```python
from build123d import *

# Parameters (mm, degrees)
ESQUISSE1_W             = 80
ESQUISSE1_H             = 80
BOSS_EXTRU_1_DEPTH      = 25
ESQUISSE2_W             = 76.4
ESQUISSE2_H             = 76.4
ENL_V_MAT_EXTRU_3_DEPTH = 22
ESQUISSE3_W             = 10
ESQUISSE3_H             = 15
ESQUISSE3_H_2           = 10
BOSS_EXTRU_2_DEPTH      = 9
ESQUISSE4_W             = 10
ESQUISSE4_H             = 10.9
ESQUISSE4_W_2           = 6
ESQUISSE4_H_2           = 10
BOSS_EXTRU_3_DEPTH      = 4
ESQUISSE5_W             = 11.2
ESQUISSE5_H             = 9.2
ESQUISSE5_W_2           = 6
ESQUISSE5_H_2           = 10.5
ENL_V_MAT_EXTRU_4_DEPTH = 10
CONG_2_R                = 2
CONG_3_R                = 1
ENL_V_MAT_EXTRU_5_DEPTH = 0.5
ENL_V_MAT_EXTRU_6_DEPTH = 0.5
ENL_V_MAT_EXTRU_7_DEPTH = 2
ENL_V_START             = -2
ENL_V_MAT_EXTRU_8_DEPTH = 2


with BuildPart() as part:
    # Esquisse1 → Boss.-Extru.1 (new body)
    with BuildSketch(Plane.XY):
        with Locations((40, 40)):
            Rectangle(ESQUISSE1_W, ESQUISSE1_H)
    extrude(amount=BOSS_EXTRU_1_DEPTH)

    # Esquisse2 → Enlèv. mat.-Extru.3 (cut)
    with BuildSketch(Plane.XY.offset(25)):
        with Locations((40.2, 40.2)):
            Rectangle(ESQUISSE2_W, ESQUISSE2_H)
    extrude(amount=-ENL_V_MAT_EXTRU_3_DEPTH, mode=Mode.SUBTRACT)

    # Esquisse3 → Boss.-Extru.2 (add)
    with BuildSketch(Plane.XY.offset(3)):
        with Locations((20, 9.5)):
            Rectangle(ESQUISSE3_W, ESQUISSE3_H)
        with Locations((73.4, 39.688534772)):
            Rectangle(ESQUISSE3_W, ESQUISSE3_H_2)
        with Locations((20, 70.9)):
            Rectangle(ESQUISSE3_W, ESQUISSE3_H)
    extrude(amount=BOSS_EXTRU_2_DEPTH)

    # Esquisse4 → Boss.-Extru.3 (add)
    with BuildSketch(Plane.XY.offset(12)):
        with Locations((20, 7.45)):
            Rectangle(ESQUISSE4_W, ESQUISSE4_H)
        with Locations((20, 72.95)):
            Rectangle(ESQUISSE4_W, ESQUISSE4_H)
        with Locations((75.4, 39.688534772)):
            Rectangle(ESQUISSE4_W_2, ESQUISSE4_H_2)
    extrude(amount=BOSS_EXTRU_3_DEPTH)

    # Esquisse5 → Enlèv. mat.-Extru.4 (cut)
    with BuildSketch(Plane.ZY):
        with Locations((19.4, 21)):
            Rectangle(ESQUISSE5_W, ESQUISSE5_H)
        with Locations((15, 33.25)):
            Rectangle(ESQUISSE5_W_2, ESQUISSE5_H_2)
    extrude(amount=-ENL_V_MAT_EXTRU_4_DEPTH, mode=Mode.SUBTRACT)

    # Congé2
    cong_2_edges = [part.edges().sort_by_distance(p)[0] for p in [
        (1, 28, 12),
        (1, 38.5, 12),
    ]]
    fillet(cong_2_edges, radius=CONG_2_R)

    # Congé3
    cong_3_edges = [part.edges().sort_by_distance(p)[0] for p in [
        (1, 38.5, 18),
        (1, 28, 18),
    ]]
    fillet(cong_3_edges, radius=CONG_3_R)

    # Esquisse8 → Enlèv. mat.-Extru.5 (cut)
    with BuildSketch(Plane.ZY):
        with BuildLine():
            add(Edge.make_bspline(
                [(7.313237468, 65.833159363), (7.48897389, 65.712447359), (7.804126252, 65.49597161), (8.487346274, 65.283616184), (8.981094379, 65.226001547), (9.307707678, 65.18788959)],
                knots=[0, 0, 0, 0, 0.299076085, 0.536340353, 1, 1, 1, 1], degree=3))
            add(Edge.make_bspline(
                [(7.284702647, 65.80245585), (7.293856567, 65.81317431), (7.303547017, 65.823166837), (7.313237468, 65.833159363)],
                knots=[0.816445355, 0.816445355, 0.816445355, 0.816445355, 1, 1, 1, 1], degree=3))
            add(Edge.make_bspline(
                [(17.901527847, 50.874632789), (17.356129628, 51.530826995), (16.293469748, 52.809362994), (15.275532925, 55.228252674), (13.933854466, 57.885340246), (11.93358483, 60.745765414), (9.727873266, 63.52670077), (8.030552607, 65.116137898), (7.284702647, 65.80245585)],
                knots=[0, 0, 0, 0, 0.134488449, 0.262038771, 0.413324325, 0.606278792, 0.814215894, 0.974718857, 0.974718857, 0.974718857, 0.974718857], degree=3))
            add(Edge.make_bspline(
                [(7.407085151, 65.469076199), (7.997724667, 64.952415937), (9.572762834, 63.532102924), (11.741354127, 60.845320938), (13.846315376, 57.844082794), (15.265007359, 55.100127721), (16.333677342, 52.722721211), (17.367018575, 51.504680356), (17.901527847, 50.874632789)],
                knots=[0.043476968, 0.043476968, 0.043476968, 0.043476968, 0.167785205, 0.379770977, 0.589080615, 0.748039182, 0.869669971, 1, 1, 1, 1], degree=3))
            add(Edge.make_bspline(
                [(7.987837686, 63.516054267), (7.933705658, 63.852405499), (7.85098554, 64.366389832), (7.741769984, 65.069503506), (7.523361561, 65.343113704), (7.407085151, 65.469076199)],
                knots=[0, 0, 0, 0, 0.449393835, 0.686726756, 0.906490115, 0.906490115, 0.906490115, 0.906490115], degree=3))
            add(Edge.make_bspline(
                [(9.581947331, 60.333994368), (9.35896114, 60.695257019), (8.925646923, 61.397274669), (8.371533969, 62.453225866), (8.111622296, 63.17317422), (7.987837686, 63.516054267)],
                knots=[0, 0, 0, 0, 0.357022344, 0.693777745, 1, 1, 1, 1], degree=3))
            add(Edge.make_bspline(
                [(9.923647007, 61.990871165), (9.797152593, 61.702831345), (9.59150409, 61.234550131), (9.533644523, 60.653068807), (9.572467818, 60.3966133), (9.581947331, 60.333994368)],
                knots=[0, 0, 0, 0, 0.547075637, 0.889409121, 1, 1, 1, 1], degree=3))
            add(Edge.make_bspline(
                [(9.845334721, 59.996400955), (9.811598018, 60.115915835), (9.717723572, 60.448473327), (9.824688072, 61.125443291), (9.886572886, 61.666645995), (9.923647007, 61.990871165)],
                knots=[0, 0, 0, 0, 0.183614026, 0.510917298, 1, 1, 1, 1], degree=3))
            add(Edge.make_bspline(
                [(12.516751585, 56.360012475), (12.220146813, 56.731946706), (11.602008437, 57.507075242), (10.696458869, 58.709807691), (10.128597293, 59.568209935), (9.845334721, 59.996400955)],
                knots=[0, 0, 0, 0, 0.316155138, 0.658882265, 1, 1, 1, 1], degree=3))
            add(Edge.make_bspline(
                [(12.5243775, 58.549530139), (12.475747631, 58.195383202), (12.389698733, 57.568732254), (12.460969789, 56.835777723), (12.504804941, 56.461905897), (12.516751585, 56.360012475)],
                knots=[0, 0, 0, 0, 0.485970736, 0.859908672, 1, 1, 1, 1], degree=3))
            add(Edge.make_bspline(
                [(12.712972257, 56.117743005), (12.689100366, 56.22919998), (12.605595842, 56.619079516), (12.538586692, 57.433441747), (12.529671109, 58.133733427), (12.5243775, 58.549530139)],
                knots=[0, 0, 0, 0, 0.139880518, 0.489305866, 1, 1, 1, 1], degree=3))
            add(Edge.make_bspline(
                [(13.853926539, 54.716920987), (13.770782279, 54.821999659), (13.560207416, 55.088126596), (13.175056735, 55.551153097), (12.879119476, 55.914019785), (12.712972257, 56.117743005)],
                knots=[0, 0, 0, 0, 0.222488299, 0.563483801, 1, 1, 1, 1], degree=3))
            add(Edge.make_bspline(
                [(18.605458509, 50.170702126), (18.280931893, 50.44303874), (17.255771256, 51.303334203), (15.614574097, 52.765406202), (14.427661827, 54.080988547), (13.853926539, 54.716920987)],
                knots=[0, 0, 0, 0, 0.193087, 0.609950563, 1, 1, 1, 1], degree=3))
            add(Edge.make_bspline(
                [(16.20036208, 54.159642546), (16.438779976, 53.603827531), (16.879859527, 52.575554733), (17.742560122, 51.269607993), (18.332407028, 50.518434698), (18.605458509, 50.170702126)],
                knots=[0, 0, 0, 0, 0.387194684, 0.716320628, 1, 1, 1, 1], degree=3))
            add(Edge.make_bspline(
                [(13.443300319, 61.775879008), (13.77418719, 60.915642263), (14.463863001, 59.122629222), (15.329762312, 56.564659638), (15.935132531, 54.892334677), (16.20036208, 54.159642546)],
                knots=[0, 0, 0, 0, 0.341315206, 0.711411851, 1, 1, 1, 1], degree=3))
            add(Edge.make_bspline(
                [(11.976778106, 61.384610882), (12.233772331, 61.501042009), (12.640271025, 61.685206075), (13.157414565, 61.862407498), (13.381058534, 61.794717609), (13.443300319, 61.775879008)],
                knots=[0, 0, 0, 0, 0.553685075, 0.875787227, 1, 1, 1, 1], degree=3))
            add(Edge.make_bspline(
                [(13.279343135, 62.10408668), (13.23692898, 62.085588167), (13.051332425, 62.004642073), (12.566317448, 61.865427123), (12.210103671, 61.574906445), (11.976778106, 61.384610882)],
                knots=[0, 0, 0, 0, 0.092717793, 0.405716039, 1, 1, 1, 1], degree=3))
            add(Edge.make_bspline(
                [(13.003343655, 62.694801827), (13.032902353, 62.635423942), (13.094815074, 62.511052886), (13.186462069, 62.313925775), (13.247594869, 62.175813112), (13.279343135, 62.10408668)],
                knots=[0, 0, 0, 0, 0.305139846, 0.639136348, 1, 1, 1, 1], degree=3))
            add(Edge.make_bspline(
                [(9.307707678, 65.18788959), (9.767844099, 65.137295561), (10.719249787, 65.03268431), (12.109364501, 64.17933924), (12.684347555, 63.224525191), (13.003343655, 62.694801827)],
                knots=[0, 0, 0, 0, 0.294280708, 0.608472459, 1, 1, 1, 1], degree=3))
        make_face()
    extrude(amount=-ENL_V_MAT_EXTRU_5_DEPTH, mode=Mode.SUBTRACT)

    # Esquisse11 → Enlèv. mat.-Extru.6 (cut)
    with BuildSketch(Plane.ZY):
        with BuildLine():
            add(Edge.make_bspline(
                [(7.243895568, 65.607536557), (7.235472734, 65.629492421), (7.214919328, 65.683069137), (7.244525992, 65.745776075), (7.269630044, 65.777003976), (7.274021635, 65.782146154)],
                knots=[0, 0, 0, 0, 0.298493917, 0.728385063, 0.816445355, 0.816445355, 0.816445355, 0.816445355], degree=3))
            add(Edge.make_bspline(
                [(7.274021635, 65.782146154), (7.156541314, 65.890249469), (7.038900997, 65.998201789), (6.921260681, 66.10615411)],
                knots=[0.974718857, 0.974718857, 0.974718857, 0.974718857, 1, 1, 1, 1], degree=3))
            add(Edge.make_bspline(
                [(6.921260681, 66.10615411), (6.831714942, 66.177342754), (6.574667912, 66.381694519), (6.223380928, 66.669125539), (5.956637647, 66.879112302), (5.858032076, 66.956736993)],
                knots=[0, 0, 0, 0, 0.25204317, 0.723506773, 1, 1, 1, 1], degree=3))
            add(Edge.make_bspline(
                [(5.858032076, 66.956736993), (5.873494425, 66.928903501), (5.924043753, 66.837910578), (6.022316687, 66.682245025), (6.087700791, 66.544864522), (6.122006074, 66.472784663)],
                knots=[0, 0, 0, 0, 0.173191566, 0.566195825, 1, 1, 1, 1], degree=3))
            add(Edge.make_bspline(
                [(6.122006074, 66.472784663), (6.149493678, 66.44984741), (6.251171186, 66.365001792), (6.467685513, 66.201886466), (6.660833558, 66.067810503), (6.774608459, 65.988832333)],
                knots=[0, 0, 0, 0, 0.132137543, 0.488780926, 1, 1, 1, 1], degree=3))
            add(Edge.make_bspline(
                [(6.774608459, 65.988832333), (6.982217829, 65.809150718), (7.189827198, 65.629469103), (7.396404139, 65.448766503)],
                knots=[0, 0, 0, 0, 0.043476968, 0.043476968, 0.043476968, 0.043476968], degree=3))
            add(Edge.make_bspline(
                [(7.396404139, 65.448766503), (7.346928222, 65.502363874), (7.295411895, 65.554950216), (7.243895568, 65.607536557)],
                knots=[0.906490115, 0.906490115, 0.906490115, 0.906490115, 1, 1, 1, 1], degree=3))
        make_face()
    extrude(amount=-ENL_V_MAT_EXTRU_6_DEPTH, mode=Mode.SUBTRACT)

    # Esquisse12 → Enlèv. mat.-Extru.7 (cut)
    with BuildSketch(Plane(origin=(0, 0, 0), x_dir=(-1, 0, 0), z_dir=(0, -1, 0))):
        with BuildLine():
            Line((-10, -20.5), (-70, -20.5))
            ThreePointArc((-70, -20.5), (-71.5, -19), (-70, -17.5))
            Line((-70, -17.5), (-10, -17.5))
            ThreePointArc((-10, -17.5), (-8.5, -19), (-10, -20.5))
        make_face()
        with BuildLine():
            Line((-70, -8.5), (-30, -8.5))
            ThreePointArc((-30, -8.5), (-28.5, -10), (-30, -11.5))
            Line((-30, -11.5), (-70, -11.5))
            ThreePointArc((-70, -11.5), (-71.5, -10), (-70, -8.5))
        make_face()
    extrude(amount=-ENL_V_MAT_EXTRU_7_DEPTH, mode=Mode.SUBTRACT)

    # Esquisse14 → Enlèv. mat.-Extru.8 (cut)
    with BuildSketch(Plane(origin=(0, 80, 0), x_dir=(1, 0, 0), z_dir=(0, 1, 0)).offset(ENL_V_START)):
        with BuildLine():
            Line((70, -20.5), (10, -20.5))
            ThreePointArc((10, -20.5), (8.5, -19), (10, -17.5))
            Line((10, -17.5), (70, -17.5))
            ThreePointArc((70, -17.5), (71.5, -19), (70, -20.5))
        make_face()
        with BuildLine():
            Line((70, -11.5), (30, -11.5))
            ThreePointArc((30, -11.5), (28.5, -10), (30, -8.5))
            Line((30, -8.5), (70, -8.5))
            ThreePointArc((70, -8.5), (71.5, -10), (70, -11.5))
        make_face()
    extrude(amount=ENL_V_MAT_EXTRU_8_DEPTH, mode=Mode.SUBTRACT)


solid = part.part
```
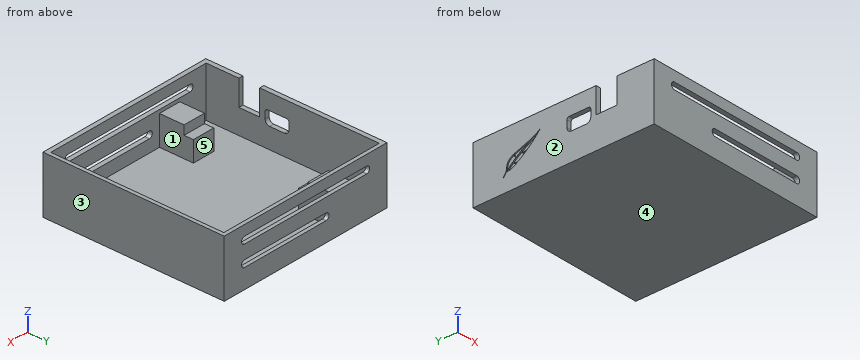
The model under review builds one solid part; all positions refer to its coordinate system, in mm. Face numbers are marked on the shaded views. A direction names the side the tool comes from. Give positions to 0.01 mm unless a question says otherwise; leave off trailing zeros. Loops run counter-clockwise (first coordinate to the right, second up) from the corner with the lowest first, then second, coordinate; pieces in that order, holes last. Notation, with made-up numbers: (41.5, -7) - (95.5, -7) arc R17 cw to (95.5, 22) - close; hole circle Ø6 at (-33.75, 79.5). An arc over 180 degrees is marked (long way). Answer as a JSON object with one key per item and string values.
Q1. For the marked faces 1 and 2, list the 3-axis set-ups (+Z, -Z, +X, -X, +Y, -Y) from which the entire face can be reached by the end or side of a thin tool; tool diameter is ignored.
Worked out:
{"face 1": "+Z", "face 2": "+Z, -Z, -X, +Y, -Y"}
Q2. Mouldability with a two-part tool opening along X and no side actions: class the marked faces 3, 4 and 5 as +X half, -X half, draft (parallel to the pull), parting line (faces both ways), or undercut.
Worked out:
{"face 3": "+X half", "face 4": "draft", "face 5": "undercut"}
Q3. Insertion check: pin 1 (3 mm diameter, centred on x = 43.5, y = 13.5, fed in from +Z); pin 2 (5 mm diameter, centred on x = 19, y = 7.5, fed in from +Z); pin 3 (1.2 mm diameter, centred on x = 22, y = 66, fed in from +Z). Each pin has a flat end and moves straight along its axis. Give the tip position at first contact, or say it passes through.
Worked out:
{"pin 1": "stops at z = 3", "pin 2": "stops at z = 16", "pin 3": "stops at z = 12"}
Q4. Add section B-B on z = 22. State the section outline as (x, y) points, plus the area to 3 significant figures.
Worked out:
{"outline": "(0, 0) - (80, 0) - (80, 80) - (0, 80) - (0, 25.6) - (2, 25.6) - (2, 78.4) - (78.4, 78.4) - (78.4, 2) - (2, 2) - (2, 16.4) - (0, 16.4) - close", "area": "545 mm^2"}
Q5. Add section C-C on x = 6. State the section outline as (y, z) points.
Worked out:
{"outline": "(0, 0) - (80, 0) - (80, 25) - (78.4, 25) - (78.4, 3) - (2, 3) - (2, 25) - (0, 25) - close"}
Q6. To check wall thickness, follow line 1 along X through (y, z) = (7.5, 12.25); line 2 along Y through (x, z) = (70, 23.25); line 3 along X through (y, z) = (35.5, 6). State the ranges of each line that lie inside material, in increasing order.
Worked out:
{"line 1": "x = 0 to 2, 15 to 25, 78.4 to 80", "line 2": "y = 0 to 2, 78.4 to 80", "line 3": "x = 0 to 2, 68.4 to 80"}
Q7. Add section A-A on x = 49. State the section outline as (y, z) points.
Worked out:
{"outline": "(0, 0) - (80, 0) - (80, 8.5) - (78.4, 8.5) - (78.4, 3) - (2, 3) - (2, 8.5) - (0, 8.5) - close; (0, 11.5) - (2, 11.5) - (2, 17.5) - (0, 17.5) - close; (0, 20.5) - (2, 20.5) - (2, 25) - (0, 25) - close; (78.4, 11.5) - (80, 11.5) - (80, 17.5) - (78.4, 17.5) - close; (78.4, 20.5) - (80, 20.5) - (80, 25) - (78.4, 25) - close"}
